Can you work these out from the drawing? Everything is in mm from the part's minimum corner. A direction names the side the tool comes from. Coordinates: 2 decimals unless noted, no trailing zeros. Loops run counter-clockwise (first coordinate to the right, second up) from the corner with the lowest first, then second, coordinate; pieces in that order, holes last. Notation, with made-up numbers: (72, 44) - (100, 44) arc R8 cw to (100, 52) - close; hole circle Ø11 at (12.25, 0.25). An arc over 180 degrees is marked (long way). Put each result on its own line as item: value. Start each with the question number.
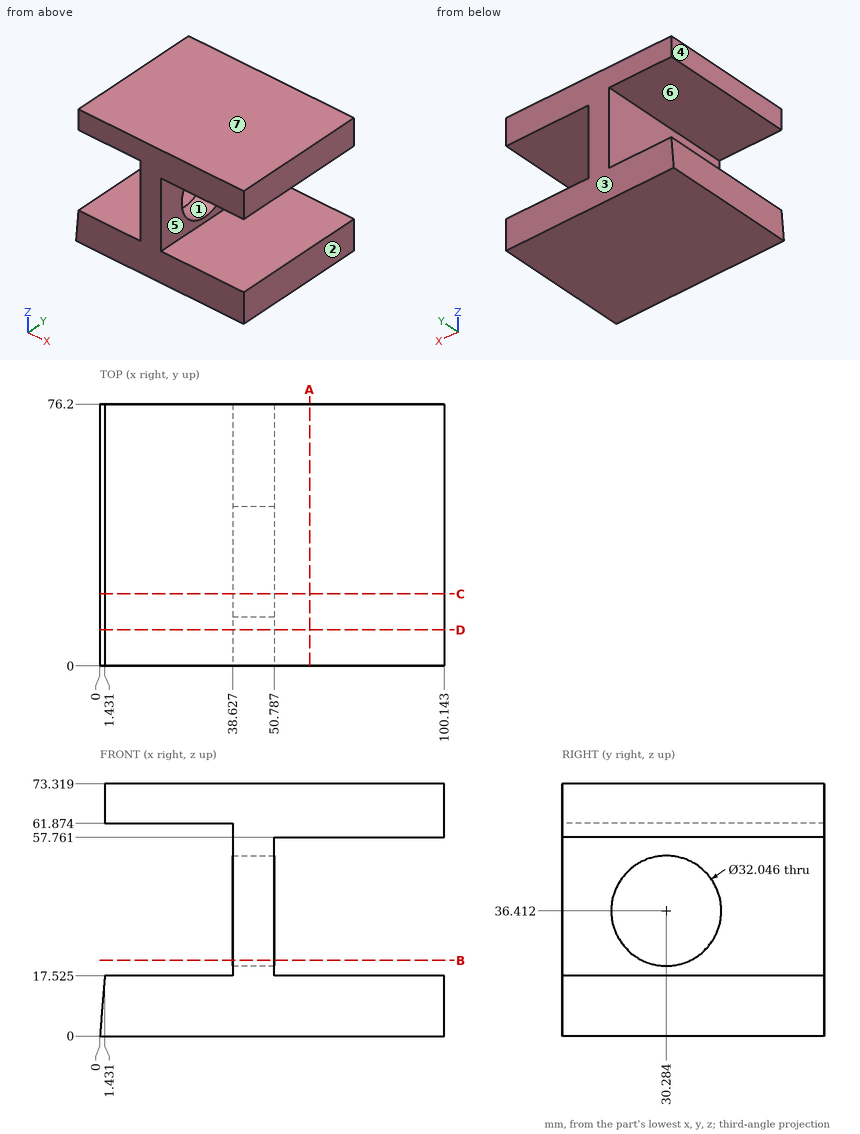
(1) I need wall thicknesses on L1, parallel to Z at x = 83, y = 41 (1 decimal); L2, parallel to Z at x = 15, y = 7.5 (1 decimal); L3, parallel to X at y = 64, z = 22.5. Which ranges of each line are inside material? Lowest first, please. Write a range as [from, to].
(2) I want a section at B-B on z = 22. List the corners of the cut face in (x, y) for me (1 decimal).
(3) I want a section at A-A on x = 61. List the corners of the cut face in (y, z) for me (1 decimal).
(4) If we mould it in two halves opening along Y, with no side actions, what happens to the marked faces 1, 2 and 3? For each: pulls with the +Y half, pulls with the -Y half, needs draft (parallel to the pull), parting line crosses it, or undercut.
(5) For pin 1 Ø8 at (y, z) = (52.5, 38.5) entering from +X; pin 2 Ø19 at (y, z) = (30.28, 36.41) entering from -X; pin 3 Ø12 at (y, z) = (61, 35.5) entering from -X; pin 4 Ø3.5 at (y, z) = (36, 66) entering from -X, each with a flat end and sliding along its axis, tell me the tip position at first contact or that it passes through.
(6) Which directions (+Z, -Z, +X, -X, +Y, -Y) give clear straight access to the entire face, cutting with the end or side of a thin tool? Please do the marked faces 4, 5, 6 and 7.
(7) I want a section at D-D on y = 10.5. List the corners of the cut face in (x, z) for me (1 decimal).
(8) I want a section at C-C on y = 21. List the corners of the cut face in (x, z) for me (1 decimal), and give its area (3 significant figures).
Answer sheet:
1. L1: z = [0, 17.5], [57.8, 73.3]
1. L2: z = [0, 17.5], [61.9, 73.3]
1. L3: x = [38.63, 50.79]
2. outline: (38.6, 0) - (50.8, 0) - (50.8, 23.3) - (38.6, 23.3) - close; (38.6, 37.3) - (50.8, 37.3) - (50.8, 76.2) - (38.6, 76.2) - close
3. outline: (0, 0) - (76.2, 0) - (76.2, 17.5) - (0, 17.5) - close; (0, 57.8) - (76.2, 57.8) - (76.2, 73.3) - (0, 73.3) - close
4. face 1: undercut
4. face 2: needs draft
4. face 3: pulls with the +Y half
5. pin 1: stops at x = 50.79
5. pin 2: passes through
5. pin 3: stops at x = 38.63
5. pin 4: stops at x = 1.43
6. face 4: +Z, -X, +Y, -Y
6. face 5: +X, +Y, -Y
6. face 6: -X, +Y, -Y
6. face 7: +Z, +X, -X, +Y, -Y
7. outline: (0, 0) - (100.1, 0) - (100.1, 17.5) - (50.8, 17.5) - (50.8, 57.8) - (100.1, 57.8) - (100.1, 73.3) - (1.4, 73.3) - (1.4, 61.9) - (38.6, 61.9) - (38.6, 17.5) - (1.4, 17.5) - close
8. outline: (0, 0) - (100.1, 0) - (100.1, 17.5) - (50.8, 17.5) - (50.8, 23.4) - (38.6, 23.4) - (38.6, 17.5) - (1.4, 17.5) - close; (1.4, 61.9) - (38.6, 61.9) - (38.6, 49.5) - (50.8, 49.5) - (50.8, 57.8) - (100.1, 57.8) - (100.1, 73.3) - (1.4, 73.3) - close
8. area: 3,300 mm^2
